Part model, mm, in its own coordinate system. Face numbers are marked on the shaded views. A direction names the side the tool comes from. Round coordinates to 2 decimals unless told otherwise and drop trailing zeros. Loops run counter-clockwise (first coordinate to the right, second up) from the corner with the lowest first, then second, coordinate; pieces in that order, holes last. Notation, with made-up numbers: M 45.5,74.25 L 68.5,74.25 A8 cw 68.5,82.25 Z; hole C 6,52.5 d7. An arc over 180 degrees is marked long. Write each question's results on one line, items separated by ' | '.
Autodesk Fusion 360 part; units mm, degrees
sketch "Sketch1" plane through (0, 0, 0) normal (0, 0, 1) x (1, 0, 0)
  line L0 (4, 6) -> (-4, 6)
  line L1 (-6, 4) -> (-6, -4)
  line L2 (-4, -6) -> (4, -6)
  line L3 (6, -4) -> (6, 4)
  line L4 (6, 6) -> (-6, -6) construction
  line L5 (-6, 6) -> (6, -6) construction
  line L6 (9, -10) -> (-9, -10)
  line L7 (-10, -9) -> (-10, 9)
  line L8 (-9, 10) -> (9, 10)
  line L9 (10, 9) -> (10, -9)
  line L10 (10, -10) -> (-10, 10) construction
  line L11 (-10, -10) -> (10, 10) construction
  circle A0 centre (10, 0) radius 1.2
  circle A1 centre (-10, 0) radius 1.2
  circle A2 centre (10, 0) radius 3.5
  circle A3 centre (-10, 0) radius 3.5
  arc A4 (-9, 10) -> (-10, 9) centre (-9, 9) ccw
  arc A5 (10, 9) -> (9, 10) centre (9, 9) ccw
  arc A6 (-10, -9) -> (-9, -10) centre (-9, -9) ccw
  arc A7 (9, -10) -> (10, -9) centre (9, -9) ccw
  arc A8 (-4, 6) -> (-6, 4) centre (-4, 4) ccw
  arc A9 (6, 4) -> (4, 6) centre (4, 4) ccw
  arc A10 (-6, -4) -> (-4, -6) centre (-4, -4) ccw
  arc A11 (4, -6) -> (6, -4) centre (4, -4) ccw
  dimension "d1" = 12
  dimension "d2" = 12
  dimension "d3" = 20
  dimension "d4" = 20
  dimension "d5" = 2.4
  dimension "d6" = 2.4
  dimension "d7" = 7
  dimension "d8" = 7
  dimension "d9" = 10
  dimension "d10" = 10
  dimension "d11" = 1
  dimension "d12" = 1
  dimension "d13" = 1
  dimension "d14" = 2
  dimension "d15" = 2
  dimension "d16" = 2
  dimension "d17" = 2
extrude "Extrude1" add sketch "Sketch1" along normal blind 2 contours L6 L7 L8 L9 A2 A3 A4 A5 A6 A7 | L9 A0 A2 | L9 A0 A2 | L7 A1 A3 | L7 A1 A3
fillet "Fillet1" radius 1 4 edges at (10, -3.5, 1) (10, 3.5, 1) (-10, 3.5, 1) (-10, -3.5, 1)
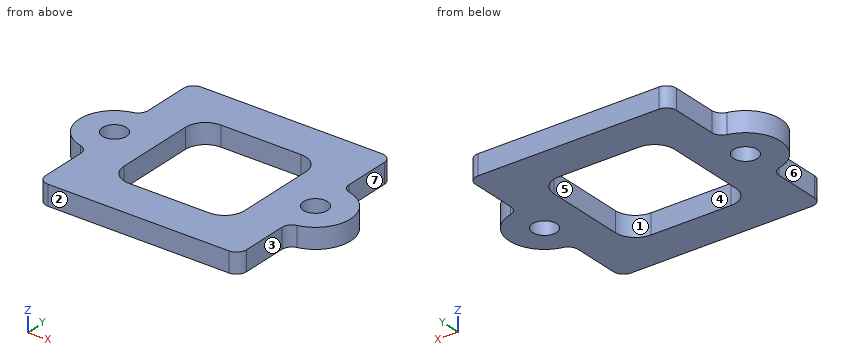
Item 1: Band-saw the part on B-B on x = 1.75. Give the cut face in (y, z), and give its area (3 significant figures).
Filled sheet:
outline: M -10,0 L -6,0 L -6,2 L -10,2 Z; M 6,0 L 10,0 L 10,2 L 6,2 Z | area: 16.0 mm^2
Item 2: Wall check: L1, parallel to Y at x = -3.5, z = 0.4; L2, parallel to X at y = -0.75, z = 0.7; L3, parallel to X at y = -0.25, z = 0.7. Give the ranges that are in metal, low to high.
Filled sheet:
L1: -10 to -6, 6 to 10 | L2: -13.42 to -10.94, -9.06 to -6, 6 to 9.06, 10.94 to 13.42 | L3: -13.49 to -11.17, -8.83 to -6, 6 to 8.83, 11.17 to 13.49
Item 3: Band-saw the part on D-D on y = 2.5. Give the cut face in (x, z).
Filled sheet:
outline: M -12.45,0 L -6,0 L -6,2 L -12.45,2 Z; M 6,0 L 12.45,0 L 12.45,2 L 6,2 Z
Item 4: Two-plate mould, pull along Y, no slides. Class the marked faces 1, 2, 3 and 4: +Y half, -Y half, draft (parallel to the pull), parting line (faces both ways), or undercut.
Filled sheet:
face 1: undercut | face 2: -Y half | face 3: draft | face 4: undercut
Item 5: Drop flat-ended pins along their axis: P1, Ø1, axis at y = -2, z = 1.5, coming from the -X side; P2, Ø0.6, axis at y = 7, z = 1, coming from the -X side. Give the stop position or say it passes through.
Filled sheet:
P1: x = -13.16 | P2: x = -10
Item 6: Band-saw the part on C-C on z = 1.15. Give the cut face in (x, y).
Filled sheet:
outline: M -10.78,-3.41 A1 cw -10,-4.39 L -10,-9 A1 ccw -9,-10 L 9,-10 A1 ccw 10,-9 L 10,-4.39 A1 cw 10.78,-3.41 A3.5 ccw 10.78,3.41 A1 cw 10,4.39 L 10,9 A1 ccw 9,10 L -9,10 A1 ccw -10,9 L -10,4.39 A1 cw -10.78,3.41 A3.5 ccw Z; hole C -10,0 d2.4; hole M -6,-4 A2 ccw -4,-6 L 4,-6 A2 ccw 6,-4 L 6,4 A2 ccw 4,6 L -4,6 A2 ccw -6,4 Z; hole C 10,0 d2.4
Item 7: Which spindle directions (+Z, -Z, +X, -X, +Y, -Y) get a long thin tool onto all of the face, cutting with end or side? Do the marked faces 5, 6 and 7. Say none if no direction does.
Filled sheet:
face 5: +Z, -Z | face 6: +Z, -Z, -X, -Y | face 7: +Z, -Z, +X, +Y
Item 8: Band-saw the part on A-A on y = 0. Give the cut face in (x, z), and give its area (3 significant figures).
Filled sheet:
outline: M -13.5,0 L -11.2,0 L -11.2,2 L -13.5,2 Z; M -8.8,0 L -6,0 L -6,2 L -8.8,2 Z; M 6,0 L 8.8,0 L 8.8,2 L 6,2 Z; M 11.2,0 L 13.5,0 L 13.5,2 L 11.2,2 Z | area: 20.4 mm^2
